Input: part model. Units: mm. Frame: model coordinates. A direction names the side the tool comes from. Round coordinates to 2 decimals unless told otherwise and drop trailing zeros. Loops run counter-clockwise (first coordinate to the right, second up) from the corner with the lowest first, then second, coordinate; pieces in that order, holes last. Notation, with made-up numbers: (72.25, 86.25) - (101.25, 86.25) arc R34 cw to (101.25, 117.25) - close; hole circle Ø4 at (-11, 78.5). An arc over 180 degrees is marked (long way). Write each question's results on one line, items separated by ' | '.
from build123d import *

# Parameters (mm, degrees)
SKETCH1_R           = 2.5
BOSS_EXTRUDE1_DEPTH = 3.5
CUT_EXTRUDE1_DEPTH  = 1.25
SKETCH3_R           = 4
SKETCH3_R_2         = 2.5
BOSS_EXTRUDE4_DEPTH = 1.25
CUT_EXTRUDE2_DEPTH  = 58.671073524
CUT_EXTRUDE3_DEPTH  = 58.671073524


with BuildPart() as part:
    # Sketch1 → Boss-Extrude1 (new, symmetric)
    with BuildSketch(Plane.XY):
        with BuildLine():
            Line((39.9669967, 0), (-30.0330033, 0))
            Line((-30.0330033, 0), (-52.420918739, 11.12570188))
            Line((-52.420918739, 11.12570188), (-52.420918739, 16.12570188))
            Line((-52.420918739, 16.12570188), (-37.420918739, 16.12570188))
            ThreePointArc((-37.420918739, 16.12570188), (-21.237684162, 14.399118341), (-7.420918739, 23))
            Line((-7.420918739, 23), (13.603539052, 23))
            Line((13.603539052, 23), (13.603539052, 20))
            ThreePointArc((13.603539052, 20), (15.068005146, 16.464466094), (18.603539052, 15))
            Line((18.603539052, 15), (39.9669967, 15))
            ThreePointArc((39.9669967, 15), (47.4669967, 7.5), (39.9669967, 0))
        make_face()
        with Locations((39.9669967, 7.5)):
            Circle(SKETCH1_R, mode=Mode.SUBTRACT)
        with Locations((9.9669967, 7.5)):
            Circle(SKETCH1_R, mode=Mode.SUBTRACT)
    extrude(amount=BOSS_EXTRUDE1_DEPTH, both=True)

    # Sketch2 → Cut-Extrude1 (cut)
    with BuildSketch(Plane.XY.offset(3.5)):
        with BuildLine():
            Line((39.9669967, 14), (18.603539052, 14))
            ThreePointArc((18.603539052, 14), (14.360898365, 15.757359313), (12.603539052, 20))
            Line((12.603539052, 20), (12.603539052, 22))
            Line((12.603539052, 22), (-6.950732305, 22))
            ThreePointArc((-6.950732305, 22), (-21.138653729, 13.396213633), (-37.641111866, 15.12570188))
            Line((-37.641111866, 15.12570188), (-51.420918739, 15.12570188))
            Line((-51.420918739, 15.12570188), (-51.420918739, 11.745424522))
            Line((-51.420918739, 11.745424522), (-29.798223995, 1))
            Line((-29.798223995, 1), (39.9669967, 1))
            ThreePointArc((39.9669967, 1), (46.4669967, 7.5), (39.9669967, 14))
        make_face()
    cut_extrude1 = extrude(amount=-CUT_EXTRUDE1_DEPTH, mode=Mode.SUBTRACT)

    # Sketch3 → Boss-Extrude4 (add)
    # profile 1 of 2: a face of its own
    with BuildSketch(Plane.XY.offset(2.25)):
        with Locations((9.9669967, 7.5)):
            Circle(SKETCH3_R)
        with Locations((9.9669967, 7.5)):
            Circle(SKETCH3_R_2, mode=Mode.SUBTRACT)
    # profile 2 of 2: a face of its own
    with BuildSketch(Plane.XY.offset(2.25)):
        with Locations((39.9669967, 7.5)):
            Circle(SKETCH3_R)
        with Locations((39.9669967, 7.5)):
            Circle(SKETCH3_R_2, mode=Mode.SUBTRACT)
    boss_extrude4 = extrude(amount=BOSS_EXTRUDE4_DEPTH)

    # Mirror1: Cut-Extrude1, Boss-Extrude4 across plane
    add(cut_extrude1.mirror(Plane.XY), mode=Mode.SUBTRACT)
    add(boss_extrude4.mirror(Plane.XY))

    # Sketch4 → Cut-Extrude2 (cut, through all)
    with BuildSketch(Plane.XY.offset(3.5)):
        Polygon((-43.37107402, 16.12570188), (-45.3835352, 16.12570188), (-44.489108009, 15.32570188), (-44.086615773, 15.32570188), align=None)
        Polygon((-41.35861284, 16.12570188), (-43.37107402, 16.12570188), (-42.476646829, 15.32570188), (-42.074154593, 15.32570188), align=None)
        Polygon((-39.34615166, 16.12570188), (-41.35861284, 16.12570188), (-40.464185649, 15.32570188), (-40.061693413, 15.32570188), align=None)
        Polygon((-37.420918739, 16.12570188), (-39.34615166, 16.12570188), (-38.451724469, 15.32570188), (-38.066677885, 15.32570188), align=None)
        Polygon((-45.3835352, 16.12570188), (-47.395996379, 16.12570188), (-46.501569188, 15.32570188), (-46.099076953, 15.32570188), align=None)
        Polygon((-47.395996379, 16.12570188), (-49.408457559, 16.12570188), (-48.514030368, 15.32570188), (-48.111538132, 15.32570188), align=None)
        Polygon((-49.408457559, 16.12570188), (-51.420918739, 16.12570188), (-50.526491548, 15.32570188), (-50.123999312, 15.32570188), align=None)
    extrude(amount=-CUT_EXTRUDE2_DEPTH, mode=Mode.SUBTRACT)

    # Sketch5 → Cut-Extrude3 (cut, through all)
    with BuildSketch(Plane.XY.offset(3.5)):
        Polygon((-4.408457559, 23), (-6.420918739, 23), (-5.642537797, 22.30379492), (-5.031162313, 22.30379492), align=None)
        Polygon((-2.395996379, 23), (-4.408457559, 23), (-3.630076617, 22.30379492), (-3.018701133, 22.30379492), align=None)
        Polygon((-0.3835352, 23), (-2.395996379, 23), (-1.617615437, 22.30379492), (-1.006239954, 22.30379492), align=None)
        Polygon((1.62892598, 23), (-0.3835352, 23), (0.394845743, 22.30379492), (1.006221226, 22.30379492), align=None)
        Polygon((3.64138716, 23), (1.62892598, 23), (2.407306922, 22.30379492), (3.018682406, 22.30379492), align=None)
        Polygon((5.65384834, 23), (3.64138716, 23), (4.419768102, 22.30379492), (5.031143586, 22.30379492), align=None)
        Polygon((7.666309519, 23), (5.65384834, 23), (6.432229282, 22.30379492), (7.043604765, 22.30379492), align=None)
        Polygon((9.678770699, 23), (7.666309519, 23), (8.444690462, 22.30379492), (9.056065945, 22.30379492), align=None)
        Polygon((11.691231879, 23), (9.678770699, 23), (10.457151641, 22.30379492), (11.068527125, 22.30379492), align=None)
        Polygon((13.603539052, 23), (11.691231879, 23), (12.469612821, 22.30379492), (12.984312686, 22.30379492), align=None)
    extrude(amount=-CUT_EXTRUDE3_DEPTH, mode=Mode.SUBTRACT)


solid = part.part
1. Contact query for flat-ended pins moving along their axis: pin 1 (3 mm diameter, centred on x = 34, y = 4.5, fed in from -Z); pin 2 (0.5 mm diameter, centred on x = -5.5, z = 1.5, fed in from +Y); pin 3 (1 mm diameter, centred on x = 21.5, z = -0.5, fed in from +Y). Output: stop coordinate, or through.
Answer:
pin 1: z = -2.25 | pin 2: y = 22.4 | pin 3: y = 15
2. Line query: line 1 (X direction, y = 7.5, z = -0.1); line 2 (X direction, y = 7, z = 0.75); line 3 (Y direction, x = 11, z = 2.75). Output: solid intervals per line, ascending. Write a range as [from, to].
Answer:
line 1: [-45.13, 7.47], [12.47, 37.47], [42.47, 47.47] | line 2: [-44.12, 7.52], [12.42, 37.52], [42.42, 47.45] | line 3: [0, 1], [3.64, 5.22], [9.78, 11.36], [22, 22.3]
3. Set-up query: faces 1 (the flat face through (-40.761, 6.448, 2.884)), 2 (the flat face through (1.5, 0.5, 3.5)), 3 (the cylindrical face through (36.79, 5.07, -2.87)), 4 (the flat face through (13.604, 22, 0)). Return all of +Z, -Z, +X, -X, +Y, -Y with unobstructed straight access to the full face (end or side cutting, diameter ignored); none if empty.
Answer:
face 1: +Z | face 2: +Z, +X, -X, +Y, -Y | face 3: -Z | face 4: +Z, -Z, +X, +Y
4. Section query B-B, the plane z = 1.25. Count the separate pieces of the cut face and the enclosed holes in it, plus the area to 3 significant figures.
Answer:
separate pieces: 1 | enclosed holes: 2 | area: 1,510 mm^2
5. Section query A-A, the plane x = 30. Output: boundary loops of the cut face in (y, z).
Answer:
outline: (0, -3.5) - (1, -3.5) - (1, -2.25) - (14, -2.25) - (14, -3.5) - (15, -3.5) - (15, 3.5) - (14, 3.5) - (14, 2.25) - (1, 2.25) - (1, 3.5) - (0, 3.5) - close
6. Section query D-D, the plane x = -32.5. Output: boundary loops of the cut face in (y, z).
Answer:
outline: (1.23, -3.5) - (2.34, -3.5) - (2.34, -2.25) - (13.4, -2.25) - (13.4, -3.5) - (14.42, -3.5) - (14.42, 3.5) - (13.4, 3.5) - (13.4, 2.25) - (2.34, 2.25) - (2.34, 3.5) - (1.23, 3.5) - close
7. Mould query, pull axis Y, two halves, no side actions, for faces 5 (the cylindrical face through (-21.46, 14.35, 0.05)), 6 (the flat face through (43, 8, -3.5)), 7 (the cylindrical face through (14.41, 15.71, -2.88)), 8 (the flat face through (-41.1, 5.5, 0)). Classes: pulls with the +Y half, pulls with the -Y half, needs draft (parallel to the pull), parting line crosses it, or undercut.
Answer:
face 5: pulls with the +Y half | face 6: needs draft | face 7: undercut | face 8: pulls with the -Y half
